Read the model definition and answer for the solid it produces. Units are mm, in the model's axes. Round coordinates to 2 decimals unless told otherwise and drop trailing zeros. Order: outer loops, then holes, each group sorted by start corner. A loop starts at its lowest first (then second) coordinate and runs counter-clockwise, first axis right, second up. Notation, with made-up numbers: (-29, 2) -> (17, 2) arc R13 ccw to (17, 26) -> close; hole circle Ø7 at (20.25, 11.25). An arc over 180 degrees is marked (long way). Use a Markdown table: item, result. Add a question column.
1. Section C-C, the plane x = 0 is taken. Give the vertices of the cut face in (y, z).
2. Section D-D, the plane x = -10 is taken. Give the vertices of the cut face in (y, z), then the cut area to 3 significant figures.
3. Section A-A, the plane z = 1.5 is taken. Give the number of separate pieces and of enclosed holes in the cut face, then the cut area to 3 significant figures.
4. Given pin 1 (3.5 mm diameter, centred on x = 0, y = -20, fed in from +Z); pin 2 (2.5 mm diameter, centred on x = 17.32, y = 10, fed in from -Z), each flat-ended and moving along its own axis, determine where each tip first touches the part or whether it passes through.
5. Section B-B, the plane y = 0 is taken. Give the vertices of the cut face in (x, z).
6. Consider L1, parallel to Y at x = 0, z = 1.1; L2, parallel to X at y = 10, z = 0.9; L3, parallel to X at y = -9, z = 0.8. Determine where each line is inside the solid, lowest interval first. Write a range as [from, to].
7. The mould has two halves that part along X. Classify faces 1 (the face through (11.5, -0.07, 1.01)), 2 (the face through (0, -6, 0)), 3 (the face through (-22.89, -7.21, 1.01)): +X half, -X half, draft (parallel to the pull), parting line (faces both ways), or undercut.
```python
from build123d import *

# Parameters (mm, degrees)
SKETCH_1_R      = 24
SKETCH_1_R_2    = 1.5
SKETCH_1_R_3    = 5
EXTRUDE_1_DEPTH = 2


with BuildPart() as part:
    # 草图1 → 凸台-拉伸1 (new body)
    with BuildSketch(Plane.XY.offset(2)):
        with Locations(Location((0, 0, 0), (0, 0, 180))):
            Circle(SKETCH_1_R)
        with Locations(Location((-17.320508076, 10, 0), (0, 0, 180))):
            Circle(SKETCH_1_R_2, mode=Mode.SUBTRACT)
        with Locations(Location((0, -20, 0), (0, 0, 180))):
            Circle(SKETCH_1_R_2, mode=Mode.SUBTRACT)
        with Locations(Location((17.320508076, 10, 0), (0, 0, 180))):
            Circle(SKETCH_1_R_2, mode=Mode.SUBTRACT)
        with Locations(Location((0, 0, 0), (0, 0, 180))):
            Circle(SKETCH_1_R_3, mode=Mode.SUBTRACT)
        with Locations(Location((0, 20, 0), (0, 0, 180))):
            Circle(SKETCH_1_R_2, mode=Mode.SUBTRACT)
        with Locations(Location((17.320508076, -10, 0), (0, 0, 180))):
            Circle(SKETCH_1_R_2, mode=Mode.SUBTRACT)
        with Locations(Location((-17.320508076, -10, 0), (0, 0, 180))):
            Circle(SKETCH_1_R_2, mode=Mode.SUBTRACT)
        with Locations(Location((0, 10, 0), (0, 0, 180))):
            Circle(SKETCH_1_R_2, mode=Mode.SUBTRACT)
        with Locations(Location((-10, 0, 0), (0, 0, 180))):
            Circle(SKETCH_1_R_2, mode=Mode.SUBTRACT)
        with Locations(Location((0, -10, 0), (0, 0, 180))):
            Circle(SKETCH_1_R_2, mode=Mode.SUBTRACT)
        with Locations(Location((10, 0, 0), (0, 0, 180))):
            Circle(SKETCH_1_R_2, mode=Mode.SUBTRACT)
    extrude(amount=-EXTRUDE_1_DEPTH)


solid = part.part
```
Verdict:
| question | item | result |
|---|---|---|
| 1 | outline | (-24, 0) -> (-21.5, 0) -> (-21.5, 2) -> (-24, 2) -> close; (-18.5, 0) -> (-11.5, 0) -> (-11.5, 2) -> (-18.5, 2) -> close; (-8.5, 0) -> (-5, 0) -> (-5, 2) -> (-8.5, 2) -> close; (5, 0) -> (8.5, 0) -> (8.5, 2) -> (5, 2) -> close; (11.5, 0) -> (18.5, 0) -> (18.5, 2) -> (11.5, 2) -> close; (21.5, 0) -> (24, 0) -> (24, 2) -> (21.5, 2) -> close |
| 2 | outline | (-21.82, 0) -> (-1.5, 0) -> (-1.5, 2) -> (-21.82, 2) -> close; (1.5, 0) -> (21.82, 0) -> (21.82, 2) -> (1.5, 2) -> close |
| 2 | area | 81.3 mm2 |
| 3 | separate pieces | 1 |
| 3 | enclosed holes | 11 |
| 3 | area | 1,660 mm2 |
| 4 | pin 1 | stops at z = 2 |
| 4 | pin 2 | passes through |
| 5 | outline | (-24, 0) -> (-11.5, 0) -> (-11.5, 2) -> (-24, 2) -> close; (-8.5, 0) -> (-5, 0) -> (-5, 2) -> (-8.5, 2) -> close; (5, 0) -> (8.5, 0) -> (8.5, 2) -> (5, 2) -> close; (11.5, 0) -> (24, 0) -> (24, 2) -> (11.5, 2) -> close |
| 6 | L1 | y = [-24, -21.5], [-18.5, -11.5], [-8.5, -5], [5, 8.5], [11.5, 18.5], [21.5, 24] |
| 6 | L2 | x = [-21.82, -18.82], [-15.82, -1.5], [1.5, 15.82], [18.82, 21.82] |
| 6 | L3 | x = [-22.25, -18.44], [-16.2, -1.12], [1.12, 16.2], [18.44, 22.25] |
| 7 | face 1 | undercut |
| 7 | face 2 | draft |
| 7 | face 3 | parting line |
